Work out the finished part from the listing and answer in its coordinate system (mm). Round coordinates to 2 decimals unless told otherwise and drop trailing zeros. Write each loop counter-clockwise with the first axis right and the second up, starting at its lowest first coordinate (ties: lowest second). Pieces come first, ordered by that corner, then holes. Notation, with made-up numbers: M 13,30 L 60,30 A26 cw 60,55 Z; hole C 63,26.5 d2. An arc over 180 degrees is marked long. One line per item, written item: value. Start each with the question number.
Q1. Find section C-C (z = 5). Write down the section's boundary in (x, y), and give its area (3 significant figures).
Q2. Find section A-A (x = 64.5). Write down the section's boundary in (y, z), and give its area (3 significant figures).
Q3. Find section B-B (y = 0.5). Count the separate pieces of the cut face and the enclosed holes in it, and give its area (3 significant figures).
Q4. Consider probe 1 along Z at (x, y) = (10.5, 0.1); probe 2 along X at (y, z) = (0.7, 36); probe 3 along X at (y, z) = (0.2, 31.5). Determine where each line is inside the solid, lowest interval first.
Q5. Given pin 1 Ø0.5 at (y, z) = (0.5, 11) entering from -X, flat-ended and moving along its own axis, determine where the tip first touches the part or whether it passes through.
from build123d import *

# Parameters (mm, degrees)
ESQUISSE1_W                = 419.5
ESQUISSE1_H                = 82
BOSS_EXTRU_1_DEPTH         = 1.5875
ESQUISSE2_W                = 5
ESQUISSE2_H                = 49
ENL_V_MAT_EXTRU_1_DEPTH    = 214.72548434
ENL_V_MAT_EXTRU_2_DEPTH    = 214.72548434
R_P_TITION_LIN_AIRE1_COUNT = 2
R_P_TITION_LIN_AIRE1_PITCH = 19.921
SYM_TRIE5_COPY_1_DEPTH     = 214.72548434
ENL_V_MAT_EXTRU_3_REACH    = 215.725
ESQUISSE5_W                = 21
ESQUISSE5_H                = 8.5
SYM_TRIE6_COPY_1_DEPTH     = 214.72548434
SYM_TRIE6_COPY_2_DEPTH     = 214.72548434
SYM_TRIE6_COPY_3_DEPTH     = 214.72548434


with BuildPart() as part:
    # Esquisse1 → Boss.-Extru.1 (new body)
    with BuildSketch(Plane(origin=(0, 0, 0), x_dir=(1, 0, 0), z_dir=(0, 1, 0))):
        Rectangle(ESQUISSE1_W, ESQUISSE1_H)
    extrude(amount=BOSS_EXTRU_1_DEPTH)

    # Esquisse2 → Enlèv. mat.-Extru.1 (cut, through all)
    with BuildSketch(Plane(origin=(0, 1.5875, 0), x_dir=(1, 0, 0), z_dir=(0, 1, 0))):
        with Locations((-207.25, 0)):
            Rectangle(ESQUISSE2_W, ESQUISSE2_H)
    enl_v_mat_extru_1 = extrude(amount=-ENL_V_MAT_EXTRU_1_DEPTH, mode=Mode.SUBTRACT)

    # Symétrie1: Enlèv. mat.-Extru.1 across plane
    add(enl_v_mat_extru_1.mirror(Plane(origin=(0, 0, 0), x_dir=(0, 0, 1), z_dir=(1, 0, 0))), mode=Mode.SUBTRACT)

    # Esquisse3 → Enlèv. mat.-Extru.2 (cut, through all)
    with BuildSketch(Plane(origin=(0, 1.5875, 0), x_dir=(1, 0, 0), z_dir=(0, 1, 0))):
        Polygon((10.25, 32.4815), (160.25, 32.481498288), (160.25, 30.281498288), (10.25, 30.2815), align=None)
    enl_v_mat_extru_2 = extrude(amount=-ENL_V_MAT_EXTRU_2_DEPTH, mode=Mode.SUBTRACT)

    # Répétition linéaire1: Enlèv. mat.-Extru.2 ×2
    with Locations(*[(0, 0, i * R_P_TITION_LIN_AIRE1_PITCH) for i in range(1, R_P_TITION_LIN_AIRE1_COUNT)]):
        add(enl_v_mat_extru_2, mode=Mode.SUBTRACT)

    # Symétrie5: Enlèv. mat.-Extru.2 across plane
    add(enl_v_mat_extru_2.mirror(Plane(origin=(0, 0, 0), x_dir=(0, 0, 1), z_dir=(1, 0, 0))), mode=Mode.SUBTRACT)

    # Symétrie5 copy 1 sketch → Symétrie5 copy 1 (cut, through all)
    with BuildSketch(Plane(origin=(0, 1.5875, 19.921), x_dir=(-1, 0, 0), z_dir=(0, 1, 0))):
        Polygon((10.25, -32.4815), (160.25, -32.481498288), (160.25, -30.281498288), (10.25, -30.2815), align=None)
    extrude(amount=-SYM_TRIE5_COPY_1_DEPTH, mode=Mode.SUBTRACT)

    # Esquisse5 → Enlèv. mat.-Extru.3 (cut, up to next)
    with BuildSketch(Plane.XZ, mode=Mode.PRIVATE) as enl_v_mat_extru_3_sk1:
        with Locations((191.75, 36.75)):
            Rectangle(ESQUISSE5_W, ESQUISSE5_H)
    enl_v_mat_extru_3_tool1 = extrude(enl_v_mat_extru_3_sk1.sketch, amount=-ENL_V_MAT_EXTRU_3_REACH, mode=Mode.PRIVATE) & part.part
    # Esquisse5 → Enlèv. mat.-Extru.3 (cut, up to next)
    with BuildSketch(Plane.XZ, mode=Mode.PRIVATE) as enl_v_mat_extru_3_sk2:
        with Locations((-191.75, 36.75)):
            Rectangle(ESQUISSE5_W, ESQUISSE5_H)
    enl_v_mat_extru_3_tool2 = extrude(enl_v_mat_extru_3_sk2.sketch, amount=-ENL_V_MAT_EXTRU_3_REACH, mode=Mode.PRIVATE) & part.part
    add(enl_v_mat_extru_3_tool1.solids().sort_by_distance((191.75, 0, 36.75))[0], mode=Mode.SUBTRACT)
    add(enl_v_mat_extru_3_tool2.solids().sort_by_distance((-191.75, 0, 36.75))[0], mode=Mode.SUBTRACT)

    # Symétrie6: Enlèv. mat.-Extru.2 across plane
    add(enl_v_mat_extru_2.mirror(Plane.XY), mode=Mode.SUBTRACT)

    # Symétrie6 copy 1 sketch → Symétrie6 copy 1 (cut, through all)
    with BuildSketch(Plane(origin=(0, 1.5875, -19.921), x_dir=(1, 0, 0), z_dir=(0, 1, 0))):
        Polygon((10.25, -32.4815), (160.25, -32.481498288), (160.25, -30.281498288), (10.25, -30.2815), align=None)
    extrude(amount=-SYM_TRIE6_COPY_1_DEPTH, mode=Mode.SUBTRACT)

    # Symétrie6 copy 2 sketch → Symétrie6 copy 2 (cut, through all)
    with BuildSketch(Plane(origin=(0, 1.5875, 0), x_dir=(-1, 0, 0), z_dir=(0, 1, 0))):
        Polygon((10.25, 32.4815), (160.25, 32.481498288), (160.25, 30.281498288), (10.25, 30.2815), align=None)
    extrude(amount=-SYM_TRIE6_COPY_2_DEPTH, mode=Mode.SUBTRACT)

    # Symétrie6 copy 3 sketch → Symétrie6 copy 3 (cut, through all)
    with BuildSketch(Plane(origin=(0, 1.5875, -19.921), x_dir=(-1, 0, 0), z_dir=(0, 1, 0))):
        Polygon((10.25, 32.4815), (160.25, 32.481498288), (160.25, 30.281498288), (10.25, 30.2815), align=None)
    extrude(amount=-SYM_TRIE6_COPY_3_DEPTH, mode=Mode.SUBTRACT)


solid = part.part
The answers:
1. outline: M -204.75,0 L 204.75,0 L 204.75,1.59 L -204.75,1.59 Z
1. area: 650 mm2
2. outline: M 0,-41 L 1.59,-41 L 1.59,-32.48 L 0,-32.48 Z; M 0,-30.28 L 1.59,-30.28 L 1.59,-12.56 L 0,-12.56 Z; M 0,-10.36 L 1.59,-10.36 L 1.59,10.36 L 0,10.36 Z; M 0,12.56 L 1.59,12.56 L 1.59,30.28 L 0,30.28 Z; M 0,32.48 L 1.59,32.48 L 1.59,41 L 0,41 Z
2. area: 116 mm2
3. separate pieces: 1
3. enclosed holes: 8
3. area: 30,900 mm2
4. probe 1: -41 to -32.48, -30.28 to -12.56, -10.36 to 10.36, 12.56 to 30.28, 32.48 to 41
4. probe 2: -209.75 to -202.25, -181.25 to 181.25, 202.25 to 209.75
4. probe 3: -209.75 to -160.25, -10.25 to 10.25, 160.25 to 209.75
5. pin 1: x = -204.75
